from build123d import *


with BuildPart() as part:
    # Sketch1 → Revolve1 (revolve)
    with BuildSketch(Plane.XY):
        with BuildLine():
            Line((12.446, 7.556707519), (12.446, 26.797))
            ThreePointArc((12.446, 26.797), (11.51606403, 29.04206403), (9.271, 29.972))
            Line((9.271, 29.972), (6.858, 29.972))
            Line((6.858, 29.972), (6.858, 40.8686))
            Line((6.858, 40.8686), (6.355531141, 56.9468))
            Line((6.355531141, 56.9468), (0, 56.9468))
            Line((0, 56.9468), (0, 0))
            ThreePointArc((0, 0), (5.504622181, 0.900649456), (10.435166667, 3.508668985))
            ThreePointArc((10.435166667, 3.508668985), (11.915602547, 5.296725955), (12.446, 7.556707519))
        make_face()
    revolve(axis=Axis((0, 56.9468, 0), (0, -1, 0)))


solid = part.part
Could you check a few things on this model? Use its own coordinates, in mm. A direction names the side the tool comes from. Give positions to 0.01 mm unless a question says otherwise; leave off trailing zeros. Order: outer loops, then holes, each group sorted by start corner. A loop starts at its lowest first (then second) coordinate and runs counter-clockwise, first axis right, second up. Notation, with made-up numbers: (-39.5, 40) - (-32.5, 40) arc R29 cw to (-32.5, 77) - close; hole circle Ø9 at (86, 35). An arc over 180 degrees is marked (long way). Return JSON: item names as keys, results as strings. Group by question number.
Q1. Will these pins go through, and if not, where does the flat tip stop? pin 1 Ø3 at (x, y) = (-1, 10) entering from -Z; pin 2 Ø12 at (x, y) = (9, 25) entering from -Z; pin 3 Ø5 at (y, z) = (33.5, -1.5) entering from +X; pin 4 Ø1 at (x, y) = (-3.5, 23) entering from +Z.
Q2. Which directions (+Z, -Z, +X, -X, +Y, -Y) give clear straight access to the entire face, cutting with the end or side of a thin tool? Please do faces 1 (the face through (-6, 29.972, -4)), 2 (the face through (-2.7, 17.31, -12.15)).
Q3. Suppose I cut it at A-A, the plane x = 0. Please give me the cut outline in (y, z) (3 decimals), and give its area (3 significant figures).
Q4. Suppose I cut it at D-D, the plane y = 46.5. Please give me the cut outline in (x, z), and give its area (3 significant figures).
Q5. Suppose I cut it at B-B, the plane z = 0. Please give me the cut outline in (x, y) (3 decimals), and give its area (3 significant figures).
Q6. Suppose I cut it at C-C, the plane y = 6. Please give me the cut outline in (x, z).
Q7. Please list where these lines run through material, in increasing order: line 1 along Z through (x, y) = (0, 24.5); line 2 along Y through (x, z) = (-9.5, -2); line 3 along Z through (x, y) = (10, 22). Write a range as [from, to].
Resolved:
{
 "1": {"pin 1": "stops at z = -12.45", "pin 2": "stops at z = -12.08", "pin 3": "stops at x = 6.86", "pin 4": "stops at z = 12.08"},
 "2": {"face 1": "+Y", "face 2": "+Y, -Y"},
 "3": {"outline": "(3.509, -10.435) arc R5.08 ccw to (7.557, -12.446) - (26.797, -12.446) arc R3.175 ccw to (29.972, -9.271) - (29.972, -6.858) - (40.869, -6.858) - (56.947, -6.356) - (56.947, 6.356) - (40.869, 6.858) - (29.972, 6.858) - (29.972, 9.271) arc R3.175 ccw to (26.797, 12.446) - (7.557, 12.446) arc R5.08 ccw to (3.509, 10.435) arc R17.272 ccw to start", "area": "1,060 mm2"},
 "4": {"outline": "circle Ø13.36 at (0, 0)", "area": "140 mm2"},
 "5": {"outline": "(-12.446, 7.557) arc R5.08 ccw to (-10.435, 3.509) arc R17.272 ccw to (10.435, 3.509) arc R5.08 ccw to (12.446, 7.557) - (12.446, 26.797) arc R3.175 ccw to (9.271, 29.972) - (6.858, 29.972) - (6.858, 40.869) - (6.356, 56.947) - (-6.356, 56.947) - (-6.858, 40.869) - (-6.858, 29.972) - (-9.271, 29.972) arc R3.175 ccw to (-12.446, 26.797) - close", "area": "1,060 mm2"},
 "6": {"outline": "circle Ø24.4 at (0, 0)"},
 "7": {"line 1": "z = [-12.45, 12.45]", "line 2": "y = [2.99, 29.94]", "line 3": "z = [-7.41, 7.41]"}
}
